Geometry check sheet. Reference: the model listing, model coordinates, mm. Face numbers are marked on the shaded views. A direction names the side the tool comes from. Coordinates: 2 decimals unless noted, no trailing zeros. Write each loop counter-clockwise with the first axis right and the second up, starting at its lowest first coordinate (ties: lowest second). Pieces come first, ordered by that corner, then holes. Notation, with made-up numbers: M 44.25,12 L 63.25,12 A34 cw 63.25,49 Z; hole C -1.5,-24.75 d1. An arc over 180 degrees is marked long. Write each question's results on one line, items separated by ' | '.
```python
from build123d import *

# Parameters (mm, degrees)
ESQUISSE1_W             = 300
ESQUISSE1_H             = 95
BOSS_EXTRU_1_DEPTH      = 5
BOSS_EXTRU_2_DEPTH      = 300
BOSS_EXTRU_3_DEPTH      = 10
ESQUISSE6_R             = 8.15
ESQUISSE6_R_2           = 5
ENL_V_MAT_EXTRU_2_DEPTH = 16
ESQUISSE7_W             = 290
ESQUISSE7_H             = 23.020862504
ENL_V_MAT_EXTRU_3_DEPTH = 30
ESQUISSE9_W             = 90
ESQUISSE9_H             = 50
ENL_V_MAT_EXTRU_4_DEPTH = 5


with BuildPart() as part:
    # Esquisse1 → Boss.-Extru.1 (new body)
    with BuildSketch(Plane.XY):
        with Locations((150, 47.5)):
            Rectangle(ESQUISSE1_W, ESQUISSE1_H)
    extrude(amount=BOSS_EXTRU_1_DEPTH)

    # Esquisse3 → Boss.-Extru.2 (add)
    with BuildSketch(Plane.ZY):
        Polygon((-15, 0), (0, 0), (0, 5), align=None)
    extrude(amount=-BOSS_EXTRU_2_DEPTH)

    # Esquisse5 → Boss.-Extru.3 (add)
    with BuildSketch(Plane.XY.offset(5)):
        Polygon((195, 95), (105, 95), (0, 95), (0, 30), (0, 0), (300, 0), (300, 30), (300, 95), align=None)
    extrude(amount=BOSS_EXTRU_3_DEPTH)

    # Esquisse6 → Enlèv. mat.-Extru.2 (cut, through all)
    with BuildSketch(Plane(origin=(0, 0, 0), x_dir=(-1, 0, 0), z_dir=(0, 0, -1))):
        with Locations((-162.7, 60)):
            Circle(ESQUISSE6_R)
        with Locations((-137.3, 60)):
            Circle(ESQUISSE6_R)
        with Locations((-180, 75)):
            Circle(ESQUISSE6_R_2)
        with Locations((-180, 45)):
            Circle(ESQUISSE6_R_2)
        with Locations((-120, 75)):
            Circle(ESQUISSE6_R_2)
        with Locations((-120, 45)):
            Circle(ESQUISSE6_R_2)
    extrude(amount=-ENL_V_MAT_EXTRU_2_DEPTH, mode=Mode.SUBTRACT)

    # Esquisse7 → Enlèv. mat.-Extru.3 (cut)
    with BuildSketch(Plane.XZ):
        with Locations((150, 16.510431252)):
            Rectangle(ESQUISSE7_W, ESQUISSE7_H)
    extrude(amount=-ENL_V_MAT_EXTRU_3_DEPTH, mode=Mode.SUBTRACT)

    # Esquisse9 → Enlèv. mat.-Extru.4 (cut)
    with BuildSketch(Plane.XY.offset(15)):
        with Locations((150, 59.36084713)):
            Rectangle(ESQUISSE9_W, ESQUISSE9_H)
    extrude(amount=-ENL_V_MAT_EXTRU_4_DEPTH, mode=Mode.SUBTRACT)


solid = part.part
```
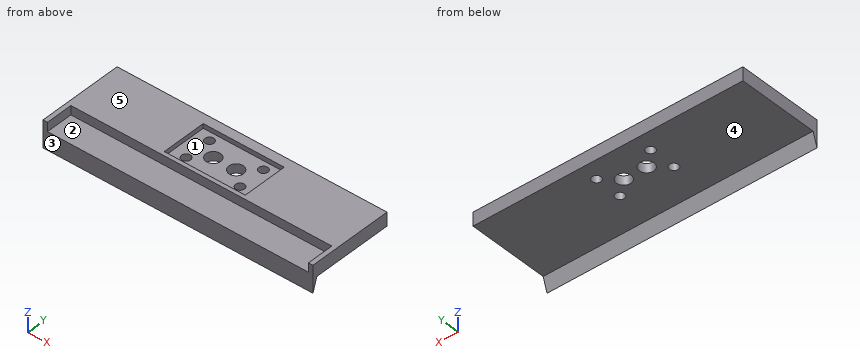
Q1. Sectioned sample at B-B on y = 45. Record the cut outline in (x, z).
Geometry check:
outline: M 0,0 L 115,0 L 115,10 L 105,10 L 105,15 L 0,15 Z; M 125,0 L 175,0 L 175,10 L 125,10 Z; M 185,0 L 300,0 L 300,15 L 195,15 L 195,10 L 185,10 Z
Q2. Access from +Z, -Z, +X, -X, +Y, -Y to the whole of each face (thin tool, end or side, straight path). Record for the marked faces 4 and 5.
Geometry check:
face 4: -Z, +X, -X, +Y | face 5: +Z, +X, -X, +Y, -Y
Q3. Sectioned sample at A-A on x = 137.3. Record the cut outline in (y, z).
Geometry check:
outline: M 0,-15 L 5,0 L 51.85,0 L 51.85,10 L 34.36,10 L 34.36,15 L 30,15 L 30,5 L 0,5 Z; M 68.15,0 L 95,0 L 95,15 L 84.36,15 L 84.36,10 L 68.15,10 Z
Q4. Mould release check, pull along X, two halves, no side actions. Record for the marked faces 1, 2 and 3: pulls with the +X half, pulls with the -X half, needs draft (parallel to the pull), parting line crosses it, or undercut.
Geometry check:
face 1: undercut | face 2: undercut | face 3: needs draft
Q5. Depth check by flat-ended pin: P1, Ø8, axis at x = 208, y = 28, coming from the -Z side; P2, Ø4, axis at x = 183.5, y = 60, coming from the +Z side; P3, Ø8, axis at x = 180, y = 45, coming from the -Z side; P4, Ø9, axis at x = 201.5, y = 17, coming from the +Z side. Enter the tip coordinate at first touch or a pass-through.
Geometry check:
P1: stops at z = 0 | P2: stops at z = 10 | P3: passes through | P4: stops at z = 5
Q6. Scan lines: probe 1 along Y at (x, z) = (120, 5.5); probe 2 along Y at (x, z) = (189.5, 10.5); probe 3 along Y at (x, z) = (162.7, 6.75). Record each from-to range of solid material in increasing order.
Geometry check:
probe 1: y = 30 to 40, 50 to 70, 80 to 95 | probe 2: y = 30 to 34.36, 84.36 to 95 | probe 3: y = 30 to 51.85, 68.15 to 95
Q7. Sectioned sample at C-C on x = 84. Record the cut outline in (y, z), and give its area (3 significant figures).
Geometry check:
outline: M 0,-15 L 5,0 L 95,0 L 95,15 L 30,15 L 30,5 L 0,5 Z | area: 1,160 mm2
Q8. Sectioned sample at D-D on y = 60. Record the cut outline in (x, z).
Geometry check:
outline: M 0,0 L 129.15,0 L 129.15,10 L 105,10 L 105,15 L 0,15 Z; M 145.45,0 L 154.55,0 L 154.55,10 L 145.45,10 Z; M 170.85,0 L 300,0 L 300,15 L 195,15 L 195,10 L 170.85,10 Z
